from build123d import *

# Parameters (mm, degrees)
F1_R          = 4.9
F2_DEPTH      = 5
F2_DEPTH_BACK = 15
F5_W          = 1.9
F5_H          = 15
F3_R          = 4.9
F7_DEPTH      = 5.001
F8_R          = 0.5
F9_DEPTH      = 5.801
F10_SIZE      = 0.2
F11_SIZE      = 0.4
F12_T1_DEPTH  = 9.6150489639
F13_SIZE      = 0.4


# Not quite as in the source:
# - a fillet or chamfer that OpenCascade refuses, or shapes differently, is made with other operations: its cross-section is extruded or revolved along the edge and cut away or added
# - a pattern or mirror of a feature is missing from the dataset's text; its kind, count and spacing are read off the source's solid


with BuildPart() as f2:
    # F1 (on Top) → F2 (new body, two sides)
    with BuildSketch(Plane.XY) as f2_sk:
        Circle(F1_R)
    extrude(amount=F2_DEPTH)
    extrude(f2_sk.sketch, amount=-F2_DEPTH_BACK)

    # F5 (on offset) → F6 (join, up to the next surface of F2)
    with BuildSketch(Plane.XZ.offset(-5.8)):
        with Locations((0, -7.5)):
            Rectangle(F5_W, F5_H)
    f6 = extrude(until=Until.NEXT)

    # F6_copies: F6 across plane
    add(f6.mirror(Plane(origin=(0, 0, 0), x_dir=(0, 0, -1), z_dir=(0, -1, 0))))

    # F3 (on Top) → F7 (cut, through all)
    with BuildSketch(Plane.XY):
        Circle(F3_R)
        with BuildLine():
            ThreePointArc((-3.5, 0), (0, 3.5), (3.5, 0))
            Line((3.5, 0), (-3.5, 0))
        make_face(mode=Mode.SUBTRACT)
    extrude(amount=F7_DEPTH, mode=Mode.SUBTRACT)

    # F8 (on face) → F9 (cut, through all)
    with BuildSketch(Plane.XZ):
        with Locations((0, 3)):
            Circle(F8_R)
    extrude(amount=-F9_DEPTH, mode=Mode.SUBTRACT)

    # F10
    f10_edges = [f2.edges().sort_by_distance(p)[0] for p in [
        (0, 3.5, 5),
        (0, 0, 5),
    ]]
    chamfer(f10_edges, length=F10_SIZE)

    # F11
    f11_edges = [f2.edges().sort_by_distance(p)[0] for p in [
        (-4.9, 0, -15),
    ]]
    chamfer(f11_edges, length=F11_SIZE)

    # F12: chamfer of 1.5 on 2 edges, made by hand

    # F12_s2 → F12_t1 (cut)
    with BuildSketch(Plane.YZ.offset(-4.8075244819)):
        Polygon((4.3, -15), (5.8, -13.5), (5.8, -15), align=None)
        Polygon((-4.3, -15), (-5.8, -13.5), (-5.8, -15), align=None)
    extrude(amount=F12_T1_DEPTH, mode=Mode.SUBTRACT)

    # F13
    f13_edges = [f2.edges().sort_by_distance(p)[0] for p in [
        (0, 5.8, 0),
        (0, -5.8, 0),
        (4.9, 0, -15),
    ]]
    chamfer(f13_edges, length=F13_SIZE)


solid = f2.part
Here's how the part is built. I have some questions about the finished solid (model axes, mm). A direction names the side the tool comes from. Coordinates: 2 decimals unless noted, no trailing zeros. Order: outer loops, then holes, each group sorted by start corner. A loop starts at its lowest first (then second) coordinate and runs counter-clockwise, first axis right, second up.
Item 1: If we section it at B-B on z = -7.5: List the corners of the cut face in (x, y) for me.
Result sheet:
outline: (-0.95, -5.8) - (0.95, -5.8) - (0.95, -4.81) arc R4.9 ccw to (0.95, 4.81) - (0.95, 5.8) - (-0.95, 5.8) - (-0.95, 4.81) arc R4.9 ccw to (-0.95, -4.81) - close
Item 2: For P1, Ø3, axis at x = -3.5, z = -8.5, coming from the +Y side; P2, Ø1.1, axis at y = -5.5, z = -8.5, coming from the -X side; P3, Ø4, axis at x = 0.5, z = 2.5, coming from the -Y side, each with a flat end and sliding along its axis, tell me the tip position at first contact or that it passes through.
Result sheet:
P1: stops at y = 4.47
P2: stops at x = -0.95
P3: stops at y = 0
Item 3: If we section it at A-A on x = 0: List the corners of the cut face in (y, z) for me.
Result sheet:
outline: (-5.8, -13.5) - (-4.3, -15) - (4.3, -15) - (5.8, -13.5) - (5.8, -0.4) - (5.4, 0) - (3.5, 0) - (3.5, 2.5) - (0, 2.5) - (0, 0) - (-5.4, 0) - (-5.8, -0.4) - close; (0, 3.5) - (3.5, 3.5) - (3.5, 4.8) - (3.3, 5) - (0.2, 5) - (0, 4.8) - close
Item 4: If we mould it in two halves opening along Z, with no side actions, what happens to faces 4 (the face through (4.61, -0.08, -14.89)), 5 (the face through (-4.9, 0.1, -7.2)), 6 (the face through (0, 1, 5)), 7 (the face through (-0.065, 1.726, 3.496))? For each: +Z half, -Z half, draft (parallel to the pull), parting line (faces both ways), or undercut.
Result sheet:
face 4: -Z half
face 5: draft
face 6: +Z half
face 7: undercut
Item 5: If we section it at C-C on z = 3: List the corners of the cut face in (x, y) for me.
Result sheet:
outline: (-3.5, 0) - (-0.5, 0) - (-0.5, 3.46) arc R3.5 ccw to start; (0.5, 0) - (3.5, 0) arc R3.5 ccw to (0.5, 3.46) - close
Item 6: For faces 1 (the face through (-0.1, 3.5, 1.8)), 2 (the face through (0, 0, 2)), 3 (the face through (-0.95, 5, -7)), which set-ups out of +Z, -Z, +X, -X, +Y, -Y let a thin tool reach every point of the face, with its end or its side?
Result sheet:
face 1: +Z, +Y
face 2: +Z, +X, -X, -Y
face 3: +Z, -Z, -X, +Y
Item 7: I need wall thicknesses on line 1 (Z direction, x = 0, y = 1.05); line 2 (X direction, y = 5, z = -10.25); line 3 (Z direction, x = -2.75, y = -1.5). Which ranges of each line are inside material? Lowest first, please.
Result sheet:
line 1: z = -15 to 2.5, 3.5 to 5
line 2: x = -0.95 to 0.95
line 3: z = -15 to 0
